For this review, take the finished solid that the model builds, in its own axes (mm). A direction names the side the tool comes from. Coordinates: 2 decimals unless noted, no trailing zeros. Write each loop counter-clockwise with the first axis right and the second up, starting at its lowest first coordinate (ties: lowest second). Pieces come first, ordered by that corner, then holes. Notation, with made-up numbers: (-8, 43) - (9, 43) arc R13 ccw to (9, 57) - close; hole circle Ø2 at (55.5, 75.5). An arc over 180 degrees is marked (long way). Write each question's results on one line, items separated by ' | '.
from build123d import *

# Parameters (mm, degrees)
SKETCH1_R           = 5.75
BOSS_EXTRUDE1_DEPTH = 3


with BuildPart() as part:
    # Sketch1 → Boss-Extrude1 (new body)
    with BuildSketch(Plane(origin=(0, 0, 0), x_dir=(1, 0, 0), z_dir=(0, 1, 0))):
        with Locations(Location((0, 0, 0), (0, 0, 270))):
            Circle(SKETCH1_R)
        with BuildLine():
            ThreePointArc((1.496877193, -0.096740213), (1.299038106, -0.75), (0.832218079, -1.247963569))
            Line((0.832218079, -1.247963569), (3.740819863, -2.927245592))
            ThreePointArc((3.740819863, -2.927245592), (2.375, -4.113620668), (0.664659115, -4.703267828))
            Line((0.664659115, -4.703267828), (0.664659115, -1.344703782))
            ThreePointArc((0.664659115, -1.344703782), (0, -1.5), (-0.664659115, -1.344703782))
            Line((-0.664659115, -1.344703782), (-0.664659115, -4.703267828))
            ThreePointArc((-0.664659115, -4.703267828), (-2.375, -4.113620668), (-3.740819863, -2.927245592))
            Line((-3.740819863, -2.927245592), (-0.832218079, -1.247963569))
            ThreePointArc((-0.832218079, -1.247963569), (-1.299038106, -0.75), (-1.496877193, -0.096740213))
            Line((-1.496877193, -0.096740213), (-4.405478977, -1.776022236))
            ThreePointArc((-4.405478977, -1.776022236), (-4.75, 0), (-4.405478977, 1.776022236))
            Line((-4.405478977, 1.776022236), (-1.496877193, 0.096740213))
            ThreePointArc((-1.496877193, 0.096740213), (-1.299038106, 0.75), (-0.832218079, 1.247963569))
            Line((-0.832218079, 1.247963569), (-3.740819863, 2.927245592))
            ThreePointArc((-3.740819863, 2.927245592), (-2.375, 4.113620668), (-0.664659115, 4.703267828))
            Line((-0.664659115, 4.703267828), (-0.664659115, 1.344703782))
            ThreePointArc((-0.664659115, 1.344703782), (0, 1.5), (0.664659115, 1.344703782))
            Line((0.664659115, 1.344703782), (0.664659115, 4.703267828))
            ThreePointArc((0.664659115, 4.703267828), (2.375, 4.113620668), (3.740819863, 2.927245592))
            Line((3.740819863, 2.927245592), (0.832218079, 1.247963569))
            ThreePointArc((0.832218079, 1.247963569), (1.299038106, 0.75), (1.496877193, 0.096740213))
            Line((1.496877193, 0.096740213), (4.405478977, 1.776022236))
            ThreePointArc((4.405478977, 1.776022236), (4.75, 0), (4.405478977, -1.776022236))
            Line((4.405478977, -1.776022236), (1.496877193, -0.096740213))
        make_face(mode=Mode.SUBTRACT)
    extrude(amount=BOSS_EXTRUDE1_DEPTH)


solid = part.part
Q1. Mouldability with a two-part tool opening along Z and no side actions: class faces 1 (the face through (-1.2, 3, 1.2)), 2 (the face through (4.85, 1.48, 3.09)), 3 (the face through (2.31, 1.48, -2.1)) as pulls with the +Z half, pulls with the -Z half, needs draft (parallel to the pull), parting line crosses it, or undercut.
Results found:
face 1: needs draft | face 2: parting line crosses it | face 3: undercut
Q2. Take a section at C-C on z = 1. State the section outline as (x, y) points, plus the area to 3 significant figures.
Results found:
outline: (-5.66, 0) - (-4.64, 0) - (-4.64, 3) - (-5.66, 3) - close; (-3.06, 0) - (-1.12, 0) - (-1.12, 3) - (-3.06, 3) - close; (1.12, 0) - (3.06, 0) - (3.06, 3) - (1.12, 3) - close; (4.64, 0) - (5.66, 0) - (5.66, 3) - (4.64, 3) - close | area: 17.8 mm2
Q3. For pin 1 (6 mm diameter, centred on x = -2.5, z = 4, fed in from -Y); pin 2 (1.5 mm diameter, centred on x = 4.5, y = 0.5, fed in from +Z); pin 3 (0.9 mm diameter, centred on y = 1.5, z = -4, fed in from -X); pin 4 (0.9 mm diameter, centred on y = 1, z = 2.5, fed in from +X), all flat-tipped, find the tip position at first contact; note any pin that passes through.
Results found:
pin 1: y = 0 | pin 2: z = 4.36 | pin 3: x = -4.52 | pin 4: x = 5.37
Q4. Take a section at A-A on x = 0. State the section outline as (y, z) points.
Results found:
outline: (0, -5.75) - (3, -5.75) - (3, -1.5) - (0, -1.5) - close; (0, 1.5) - (3, 1.5) - (3, 5.75) - (0, 5.75) - close
Q5. Wall thickness on line 1 along X through (y, z) = (1.7, 3); line 2 along X through (y, z) = (2.5, 4.25); line 3 along Z through (x, y) = (1, 1.55): over which ranges is each line inside the solid? List them lowest first. Write a range as from..to.
Results found:
line 1: -4.91..-3.68, -0.66..0.66, 3.68..4.91 | line 2: -3.87..-2.12, -0.66..0.66, 2.12..3.87 | line 3: -5.66..-4.64, -1.34..-1.12, 1.12..1.34, 4.64..5.66
Q6. Take a section at D-D on x = -2. State the section outline as (y, z) points, plus the area to 3 significant figures.
Results found:
outline: (0, -5.39) - (3, -5.39) - (3, -4.31) - (0, -4.31) - close; (0, -1.92) - (3, -1.92) - (3, -0.39) - (0, -0.39) - close; (0, 0.39) - (3, 0.39) - (3, 1.92) - (0, 1.92) - close; (0, 4.31) - (3, 4.31) - (3, 5.39) - (0, 5.39) - close | area: 15.7 mm2
Q7. For faces 4 (the face through (-1.2, 0, 1.2)), 5 (the face through (-0.665, 1, -3)), list the 3-axis set-ups (+Z, -Z, +X, -X, +Y, -Y) from which the entire face can be reached by the end or side of a thin tool; tool diameter is ignored.
Results found:
face 4: +Z, -Z, +X, -X, -Y | face 5: +Y, -Y
Q8. Take a section at B-B on y = 2.7. State the section outline as (x, z) points.
Results found:
outline: circle Ø11.5 at (0, 0); hole (-4.41, -1.78) - (-1.5, -0.1) arc R1.5 ccw to (-0.83, -1.25) - (-3.74, -2.93) arc R4.75 ccw to (-0.66, -4.7) - (-0.66, -1.34) arc R1.5 ccw to (0.66, -1.34) - (0.66, -4.7) arc R4.75 ccw to (3.74, -2.93) - (0.83, -1.25) arc R1.5 ccw to (1.5, -0.1) - (4.41, -1.78) arc R4.75 ccw to (4.41, 1.78) - (1.5, 0.1) arc R1.5 ccw to (0.83, 1.25) - (3.74, 2.93) arc R4.75 ccw to (0.66, 4.7) - (0.66, 1.34) arc R1.5 ccw to (-0.66, 1.34) - (-0.66, 4.7) arc R4.75 ccw to (-3.74, 2.93) - (-0.83, 1.25) arc R1.5 ccw to (-1.5, 0.1) - (-4.41, 1.78) arc R4.75 ccw to start
